```python
from build123d import *
from build123d.topology import SkipClean

# Parameters (mm, degrees)
SKETCH1_R      = 4.1
SKETCH1_R_2    = 1.7
EXTRUDE1_DEPTH = 0.9
EXTRUDE2_START = 7.7
SKETCH2_R      = 17.5
EXTRUDE2_DEPTH = 7.7
SKETCH3_R      = 5
EXTRUDE3_DEPTH = 1.5
SKETCH4_R      = 3.25
EXTRUDE4_DEPTH = 5.7
EXTRUDE5_DEPTH = 5.9


with BuildPart() as part:
    # Sketch1 → Extrude1 (new body)
    # profile 1 of 8: a face of its own
    with BuildSketch(Plane(origin=(0, 0, 0), x_dir=(1, 0, 0), z_dir=(0, 1, 0))):
        with BuildLine():
            ThreePointArc((-9.513184584, -14.688407642), (-17.5, 0), (-9.513184584, 14.688407642))
            Line((-9.513184584, 14.688407642), (-26.878803245, 3.441284076))
            ThreePointArc((-26.878803245, 3.441284076), (-22.691441002, 3.601950396), (-20.55, 0))
            ThreePointArc((-20.55, 0), (-22.691441002, -3.601950396), (-26.878803245, -3.441284076))
            Line((-26.878803245, -3.441284076), (-9.513184584, -14.688407642))
        make_face()
    # profile 2 of 8: a face of its own
    with BuildSketch(Plane(origin=(0, 0, 0), x_dir=(1, 0, 0), z_dir=(0, 1, 0))):
        with Locations((-24.65, 0)):
            Circle(SKETCH1_R)
        with Locations(Location((-24.65, 0, 0), (0, 0, 270))):
            Circle(SKETCH1_R_2, mode=Mode.SUBTRACT)
    # profile 3 of 8: a face of its own
    with BuildSketch(Plane(origin=(0, 0, 0), x_dir=(1, 0, 0), z_dir=(0, 1, 0))):
        with BuildLine():
            ThreePointArc((9.513184584, 14.688407642), (4.959983178, 16.782388593), (0, 17.5))
            Line((0, 17.5), (0, -17.5))
            ThreePointArc((0, -17.5), (4.959983178, -16.782388593), (9.513184584, -14.688407642))
            ThreePointArc((9.513184584, -14.688407642), (15.374178518, -8.359703038), (17.5, 0))
            ThreePointArc((17.5, 0), (15.374178518, 8.359703038), (9.513184584, 14.688407642))
        make_face()
    # profile 4 of 8: a face of its own
    with BuildSketch(Plane(origin=(0, 0, 0), x_dir=(1, 0, 0), z_dir=(0, 1, 0))):
        with BuildLine():
            Line((0, -17.5), (0, 17.5))
            ThreePointArc((0, 17.5), (-4.959983178, 16.782388593), (-9.513184584, 14.688407642))
            ThreePointArc((-9.513184584, 14.688407642), (-17.5, 0), (-9.513184584, -14.688407642))
            ThreePointArc((-9.513184584, -14.688407642), (-4.959983178, -16.782388593), (0, -17.5))
        make_face()
    # profile 5 of 8: a face of its own
    with BuildSketch(Plane(origin=(0, 0, 0), x_dir=(1, 0, 0), z_dir=(0, 1, 0))):
        with BuildLine():
            ThreePointArc((9.513184584, 14.688407642), (4.959983178, 16.782388593), (0, 17.5))
            Line((0, 17.5), (0, -17.5))
            ThreePointArc((0, -17.5), (4.959983178, -16.782388593), (9.513184584, -14.688407642))
            ThreePointArc((9.513184584, -14.688407642), (15.374178518, -8.359703038), (17.5, 0))
            ThreePointArc((17.5, 0), (15.374178518, 8.359703038), (9.513184584, 14.688407642))
        make_face()
    # profile 6 of 8: a face of its own
    with BuildSketch(Plane(origin=(0, 0, 0), x_dir=(1, 0, 0), z_dir=(0, 1, 0))):
        with BuildLine():
            Line((0, -17.5), (0, 17.5))
            ThreePointArc((0, 17.5), (-4.959983178, 16.782388593), (-9.513184584, 14.688407642))
            ThreePointArc((-9.513184584, 14.688407642), (-17.5, 0), (-9.513184584, -14.688407642))
            ThreePointArc((-9.513184584, -14.688407642), (-4.959983178, -16.782388593), (0, -17.5))
        make_face()
    # profile 7 of 8: a face of its own
    with BuildSketch(Plane(origin=(0, 0, 0), x_dir=(1, 0, 0), z_dir=(0, 1, 0))):
        with BuildLine():
            Line((26.878803245, 3.441284076), (9.513184584, 14.688407642))
            ThreePointArc((9.513184584, 14.688407642), (15.374178518, 8.359703038), (17.5, 0))
            ThreePointArc((17.5, 0), (15.374178518, -8.359703038), (9.513184584, -14.688407642))
            Line((9.513184584, -14.688407642), (26.878803245, -3.441284076))
            ThreePointArc((26.878803245, -3.441284076), (20.55, 0), (26.878803245, 3.441284076))
        make_face()
    # profile 8 of 8: a face of its own
    with BuildSketch(Plane(origin=(0, 0, 0), x_dir=(1, 0, 0), z_dir=(0, 1, 0))):
        with Locations((24.65, 0)):
            Circle(SKETCH1_R)
        with Locations(Location((24.65, 0, 0), (0, 0, 270))):
            Circle(SKETCH1_R_2, mode=Mode.SUBTRACT)
    extrude(amount=EXTRUDE1_DEPTH)

    # Sketch2 → Extrude2 (add)
    with SkipClean():  # the faces are left unmerged after this step: merging them gives an invalid solid
        with BuildSketch(Plane.XZ.offset(EXTRUDE2_START)):
            with Locations(Location((0, 0, 0), (0, 0, 270))):
                Circle(SKETCH2_R)
        extrude(amount=-EXTRUDE2_DEPTH)

    # Sketch3 → Extrude3 (add)
    with SkipClean():  # the faces are left unmerged after this step: merging them gives an invalid solid
        with BuildSketch(Plane(origin=(0, 0.9, 0), x_dir=(1, 0, 0), z_dir=(0, 1, 0))):
            with Locations(Location((0, 0, 0), (0, 0, 270))):
                Circle(SKETCH3_R)
        extrude(amount=EXTRUDE3_DEPTH)

    # Sketch4 → Extrude4 (add)
    with SkipClean():  # the faces are left unmerged after this step: merging them gives an invalid solid
        with BuildSketch(Plane(origin=(0, 2.4, 0), x_dir=(1, 0, 0), z_dir=(0, 1, 0))):
            with Locations(Location((0, 0, 0), (0, 0, 270))):
                Circle(SKETCH4_R)
        extrude(amount=EXTRUDE4_DEPTH)

    # Sketch5 → Extrude5 (add)
    with BuildSketch(Plane.XZ.offset(7.7)):
        Polygon((7.284924369, 15.911627099), (15.911627099, 7.284924369), (18.457211511, 11.3861437), (11.3861437, 18.457211511), align=None)
    extrude(amount=-EXTRUDE5_DEPTH)


solid = part.part
```
Part model, mm, in its own coordinate system. A direction names the side the tool comes from. Coordinates: 2 decimals unless noted, no trailing zeros. Loops run counter-clockwise (first coordinate to the right, second up) from the corner with the lowest first, then second, coordinate; pieces in that order, holes last. Notation, with made-up numbers: (67, -36) - (108, -36) arc R11 ccw to (108, -19) - close; hole circle Ø5 at (-2.75, 59). An arc over 180 degrees is marked (long way). Write item = value, one per line. Start each with the question number.
Item 1: Cut at A-A, the plane z = 0. Give the cut face in (x, y).
Item 2: 3-axis set-ups, long thin cutter, end or side, ignore diameter. For faces 5 (the flat face through (-18.318, 0.444, 8.986)), 6 (the cylindrical face through (-4.88, 1.64, -1.08)), 7 (the flat face through (9.36, -4.79, 17.2)), 8 (the flat face through (17.17, -4.79, 9.31)), 9 (the cylindrical face through (-28.75, 0.44, -0.06)): which of +Z, -Z, +X, -X, +Y, -Y reach the whole face in a straight line?
Item 3: Cut at D-D, the plane z = -6. Give the cut face in (x, y), and give its area (3 significant figures).
Item 4: Cut at C-C, the plane y = -6.5. Give the cut face in (x, z), and give its area (3 significant figures).
Item 5: Flat gauge pins, fed straight in: pin 1 Ø1.5 at (y, z) = (-2, -8.5) entering from -X; pin 2 Ø2 at (x, y) = (-5.5, 1.5) entering from +Z; pin 3 Ø3.5 at (x, z) = (12.5, 15.5) entering from +Y. Where does each tip first touch, or does it go through?
Item 6: Mould opens along Y. For faces 1 (the flat face through (1, -7.7, 1)), 2 (the flat face through (6, 0.9, 0)), 3 (the flat face through (18.074, 0.444, 9.144)), 4 (the flat face through (13, -1.8, 14)) say: released by +Y, released by -Y, zero draft, split by the parting line, or undercut.
Item 7: Cut at B-B, the plane x = -24.65. Give the cut face in (y, z), and give its area (3 significant figures).
Item 8: Wall check: L1, parallel to X at y = 0.65, z = 0; L2, parallel to Y at x = 22, z = 5; L3, parallel to Y at x = 2.5, z = -12. Give the ranges that are in metal, low to high. Write a range as from..to.
The answers:
q1.outline = (-28.75, 0) - (-26.35, 0) - (-26.35, 0.9) - (-28.75, 0.9) - close; (-22.95, 0) - (-17.5, 0) - (-17.5, -7.7) - (17.5, -7.7) - (17.5, 0) - (22.95, 0) - (22.95, 0.9) - (5, 0.9) - (5, 2.4) - (3.25, 2.4) - (3.25, 8.1) - (-3.25, 8.1) - (-3.25, 2.4) - (-5, 2.4) - (-5, 0.9) - (-22.95, 0.9) - close; (26.35, 0) - (28.75, 0) - (28.75, 0.9) - (26.35, 0.9) - close
q2.face_5 = +Z, -X, +Y, -Y
q2.face_6 = +Y
q2.face_7 = +Z, +Y, -Y
q2.face_8 = +X, -Y
q2.face_9 = -X, +Y, -Y
q3.outline = (-22.93, 0) - (-16.44, 0) - (-16.44, -7.7) - (16.44, -7.7) - (16.44, 0) - (22.93, 0) - (22.93, 0.9) - (-22.93, 0.9) - close
q3.area = 294 mm2
q4.outline = (7.28, 15.91) arc R17.5 ccw (long way) to (15.91, 7.28) - (18.46, 11.39) - (11.39, 18.46) - close
q4.area = 1,010 mm2
q5.pin_1 = -15.69
q5.pin_2 = 16.86
q5.pin_3 = -1.8
q6.face_1 = released by -Y
q6.face_2 = released by +Y
q6.face_3 = zero draft
q6.face_4 = undercut
q7.outline = (0, -4.88) - (0.9, -4.88) - (0.9, -1.7) - (0, -1.7) - close; (0, 1.7) - (0.9, 1.7) - (0.9, 4.88) - (0, 4.88) - close
q7.area = 5.73 mm2
q8.L1 = -28.75..-26.35, -22.95..22.95, 26.35..28.75
q8.L2 = 0..0.9
q8.L3 = -7.7..0.9
